Verification items for the finished model (mm, model axes). A direction names the side the tool comes from. Coordinates: 2 decimals unless noted, no trailing zeros. Order: outer loops, then holes, each group sorted by start corner. A loop starts at its lowest first (then second) coordinate and runs counter-clockwise, first axis right, second up.
Q1. Depth check by flat-ended pin: P1, Ø5, axis at x = 45, y = -18.5, coming from the +Z side; P2, Ø6, axis at x = 8.5, y = -12, coming from the -Z side; P3, Ø1.7, axis at y = -16, z = 20.5, coming from the +X side; P4, Ø4, axis at y = -10, z = 13.5, coming from the +X side. Enter the tip coordinate at first touch or a pass-through.
Q2. Set-up check for faces 1 (the flat face through (18.868, -13, 20)), 2 (the flat face through (18, -13, 21.414)), 3 (the flat face through (22, 0, 11)): record each of +Z, -Z, +X, -X, +Y, -Y from which the full face is reachable in a straight line by a thin tool's end or side.
Q3. Cross-section at D-D, the plane y = -9. Count the separate pieces of the cut face and the enclosed holes in it, and give its area (3 significant figures).
Q4. Cross-section at A-A, the plane y = -15.5. Record the boundary of the cut face in (x, z), and give its area (3 significant figures).
Q5. Cross-section at B-B, the plane z = 20. Record the boundary of the cut face in (x, y).
Q6. Cross-section at C-C, the plane x = 6.5. Record the boundary of the cut face in (y, z).
Q7. Thickness scan on line 1 (X direction, y = -9.25, z = 15); line 2 (Z direction, x = 17.5, y = -22); line 3 (Y direction, x = 32, z = 3). Record the ranges inside material, lowest first.
Q8. Draft check along X on faces 4 (the cylindrical face through (54.006, -12.009, 9.782)), 5 (the flat face through (0, -13, 11)), 6 (the cylindrical face through (11.378, -8.656, 23.735)). Enter one of: pulls with the +X half, pulls with the -X half, needs draft (parallel to the pull), parting line crosses it, or undercut.
from build123d import *

# Parameters (mm, degrees)
F1_DEPTH = 25.4
F2_W     = 18.867608
F2_H     = 25.4
F2_R     = 7.749335
F3_DEPTH = 25.4
F5_DEPTH = 25.4
F7_DEPTH = 25.4
F8_R     = 4.539573
F9_DEPTH = 50.8


with BuildPart() as f1:
    # F0 (on Front) → F1 (new body)
    with BuildSketch(Plane.XZ):
        Polygon((0, 46.81436), (0, 0), (55.1842, 0), (55.1842, 19.293191), (18.867608, 19.293191), (18.867608, 46.81436), align=None)
    extrude(amount=F1_DEPTH)

    # F2 (on face) → F3 (cut)
    with BuildSketch(Plane.XY.offset(46.81436)):
        with Locations((9.433804, -12.7)):
            Rectangle(F2_W, F2_H)
        with Locations((8.937289, -12.483831)):
            Circle(F2_R, mode=Mode.SUBTRACT)
    extrude(amount=-F3_DEPTH, mode=Mode.SUBTRACT)

    # F4 (on face) → F5 (cut)
    with BuildSketch(Plane.XY.offset(19.293191)):
        with BuildLine():
            ThreePointArc((44.970158, 0), (54.020374, -12.23415), (46.388779, -25.4))
            Line((46.388779, -25.4), (55.1842, -25.4))
            Line((55.1842, -25.4), (55.1842, 0))
            Line((55.1842, 0), (44.970158, 0))
        make_face()
    extrude(amount=-F5_DEPTH, mode=Mode.SUBTRACT)

    # F6 (on face) → F7 (cut)
    with BuildSketch(Plane.XY.offset(19.293191)):
        with BuildLine():
            add(Edge.make_bspline(
                [(43.551542, -10.781489), (43.551542, -4.311831), (27.379308, -7.54666), (11.207074, -10.781489), (27.379308, -14.016319), (43.551542, -17.251148), (43.551542, -10.781489)],
                knots=[0, 0, 0, 2.094395, 2.094395, 4.18879, 4.18879, 6.283185, 6.283185, 6.283185], degree=2, weights=[1, 0.5, 1, 0.5, 1, 0.5, 1]))
        make_face()
    extrude(amount=-F7_DEPTH, mode=Mode.SUBTRACT)

    # F8 (on face) → F9 (cut)
    with BuildSketch(Plane.XY.offset(46.81436)):
        with Locations((8.937289, -12.483831)):
            Circle(F8_R)
    extrude(amount=-F9_DEPTH, mode=Mode.SUBTRACT)


solid = f1.part
Check values:
1. P1: stops at z = 19.29
1. P2: passes through
1. P3: stops at x = 18.87
1. P4: stops at x = 54.01
2. face 1: +Z, +X, +Y, -Y
2. face 2: +Z
2. face 3: +Z, -Z, +X, -X, +Y
3. separate pieces: 3
3. enclosed holes: 0
3. area: 785 mm2
4. outline: (0, 0) - (5.54, 0) - (5.54, 46.81) - (1.8, 46.81) - (1.8, 21.41) - (0, 21.41) - close; (12.33, 0) - (53.82, 0) - (53.82, 19.29) - (18.87, 19.29) - (18.87, 21.41) - (16.08, 21.41) - (16.08, 46.81) - (12.33, 46.81) - close
4. area: 1,120 mm2
5. outline: (0, -25.4) - (18.87, -25.4) - (18.87, 0) - (0, 0) - close; hole circle Ø9.08 at (8.94, -12.48)
6. outline: (-25.4, 0) - (-16.31, 0) - (-16.31, 46.81) - (-19.84, 46.81) - (-19.84, 21.41) - (-25.4, 21.41) - close; (-8.65, 0) - (0, 0) - (0, 21.41) - (-5.13, 21.41) - (-5.13, 46.81) - (-8.65, 46.81) - close
7. line 1: x = 0 to 5.75, 12.12 to 22.94, 42.6 to 53.52
7. line 2: z = 0 to 21.41
7. line 3: y = -25.4 to -14.51, -7.06 to 0
8. face 4: pulls with the +X half
8. face 5: pulls with the -X half
8. face 6: undercut
